Can you work these out from the model? Positions are in its coordinate system, mm. Face numbers are marked on the shaded views. A direction names the side the tool comes from. Give positions to 0.01 mm unless a question says otherwise; leave off trailing zeros. Write each loop counter-clockwise with the first axis right and the second up, starting at its lowest first coordinate (ties: lowest second). Pieces come first, ordered by that corner, then holes.
1. Thinking about a two-plate mould opening in X: for the marked faces 3, 4 and 5, which applies, pulls with the +X half, pulls with the -X half, needs draft (parallel to the pull), parting line crosses it, or undercut?
2. Suppose I cut it at D-D (x = 90). Please give me the cut outline in (y, z).
3. Suppose I cut it at C-C (z = -2). Give the number of separate pieces and of enclosed holes in the cut face, and give its area (3 significant figures).
4. I'm going to push flat-ended pins straight in: pin 1 (3 mm diameter, centred on x = 32.5, z = -7.5, fed in from -Y); pin 2 (1.5 mm diameter, centred on x = 88.5, y = -19, fed in from +Z); pin 3 (1 mm diameter, centred on y = -14.5, z = 15, fed in from +X); pin 4 (16 mm diameter, centred on x = 90, z = 0, fed in from +Y). Where does each tip first touch, or does it pass through?
5. On a 3-axis mill with a long thin cutter (end or side, diameter ignored), from which of +Z, -Z, +X, -X, +Y, -Y can I reach the whole of each face in a straight line? I mean the marked faces 1 and 2. Say none if no direction works.
6. Suppose I cut it at A-A (y = -17.5). Please give me the cut outline in (x, z), and give its area (3 significant figures).
7. If I drill on probe 1 along Z at (x, y) = (0, -50); probe 2 along Z at (x, y) = (0, -14.5); probe 3 along X at (y, z) = (-4.5, 3.5), over which ranges is the centre line in solid material (lowest first)?
8. Suppose I cut it at B-B (x = 0). Please give me the cut outline in (y, z).
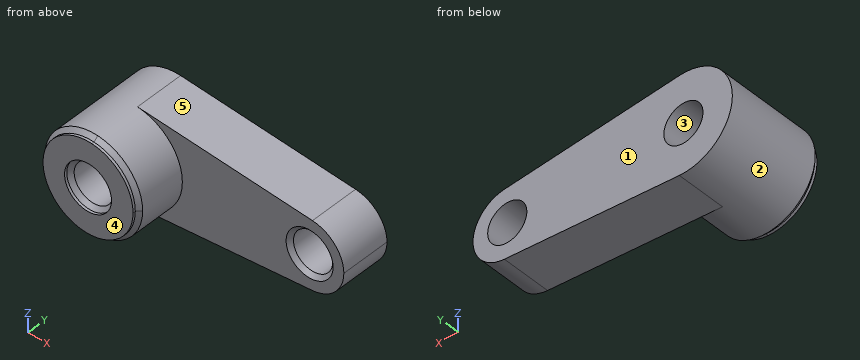
```python
from build123d import *

# Parameters (mm, degrees)
F0_R     = 10
F1_DEPTH = 25
F2_DEPTH = 50
F3_SIZE  = 2
F4_DEPTH = 1.3


with BuildPart() as f1:
    # F0 (on Front) → F1 (new body)
    with BuildSketch(Plane.XZ):
        with BuildLine():
            ThreePointArc((2.0833333333, -24.9130432148), (18.3995018048, -16.9250800097), (25, 0))
            ThreePointArc((25, 0), (18.3995018048, 16.9250800097), (2.0833333333, 24.9130432148))
            ThreePointArc((2.0833333333, 24.9130432148), (-25, 0), (2.0833333333, -24.9130432148))
        make_face()
        Circle(F0_R, mode=Mode.SUBTRACT)
        with BuildLine():
            ThreePointArc((2.0833333333, 24.9130432148), (18.3995018048, 16.9250800097), (25, 0))
            ThreePointArc((25, 0), (18.3995018048, -16.9250800097), (2.0833333333, -24.9130432148))
            Line((2.0833333333, -24.9130432148), (91.4583333333, -17.4391302504))
            ThreePointArc((91.4583333333, -17.4391302504), (72.5, 0), (91.4583333333, 17.4391302504))
            Line((91.4583333333, 17.4391302504), (2.0833333333, 24.9130432148))
        make_face()
        with BuildLine():
            ThreePointArc((107.5, 0), (102.8796512634, 11.8475560068), (91.4583333333, 17.4391302504))
            ThreePointArc((91.4583333333, 17.4391302504), (72.5, 0), (91.4583333333, -17.4391302504))
            ThreePointArc((91.4583333333, -17.4391302504), (102.8796512634, -11.8475560068), (107.5, 0))
        make_face()
        with Locations((90, 0)):
            Circle(F0_R, mode=Mode.SUBTRACT)
    extrude(amount=F1_DEPTH)

    # F0 (on Front) → F2 (join)
    with BuildSketch(Plane.XZ):
        with BuildLine():
            ThreePointArc((2.0833333333, -24.9130432148), (18.3995018048, -16.9250800097), (25, 0))
            ThreePointArc((25, 0), (18.3995018048, 16.9250800097), (2.0833333333, 24.9130432148))
            ThreePointArc((2.0833333333, 24.9130432148), (-25, 0), (2.0833333333, -24.9130432148))
        make_face()
        Circle(F0_R, mode=Mode.SUBTRACT)
    extrude(amount=F2_DEPTH)

    # F3
    f3_edges = [f1.edges().sort_by_distance(p)[0] for p in [
        (-2.083333, -50, 24.913043),
        (-10, -50, 0),
        (80, -25, 0),
    ]]
    chamfer(f3_edges, length=F3_SIZE)

    # F4 (add): a face of the model
    f4_faces = [f1.faces().sort_by_distance(p)[0] for p in [
        (-1.8624551468, -50, 22.2717242675),
    ]]
    extrude(f4_faces, amount=F4_DEPTH)


solid = f1.part
```
Checks:
1. face 3: undercut
1. face 4: needs draft
1. face 5: pulls with the +X half
2. outline: (-25, -17.56) - (0, -17.56) - (0, -10) - (-23, -10) - (-25, -12) - close; (-25, 12) - (-23, 10) - (0, 10) - (0, 17.56) - (-25, 17.56) - close
3. separate pieces: 3
3. enclosed holes: 0
3. area: 3,100 mm2
4. pin 1: stops at y = -25
4. pin 2: stops at z = 17.75
4. pin 3: stops at x = 99.8
4. pin 4: passes through
5. face 1: +Z, -Z, +X, -X, +Y
5. face 2: -Y
6. outline: (2.08, -24.91) - (91.46, -17.44) arc R17.5 ccw to (91.46, 17.44) - (2.08, 24.91) arc R25 ccw (long way) to start; hole circle Ø20 at (0, 0); hole circle Ø20 at (90, 0)
6. area: 4,670 mm2
7. probe 1: z = -23 to -12, 12 to 23
7. probe 2: z = -25 to -10, 10 to 25
7. probe 3: x = -24.75 to -9.37, 9.37 to 80.63, 99.37 to 107.15
8. outline: (-51.3, -23) - (-50, -23) - (-48, -25) - (0, -25) - (0, -10) - (-48, -10) - (-50, -12) - (-51.3, -12) - close; (-51.3, 12) - (-50, 12) - (-48, 10) - (0, 10) - (0, 25) - (-48, 25) - (-50, 23) - (-51.3, 23) - close
